Could you check a few things on this drawing? It's one solid part, dimensions in mm from its lowest x, y, z. A direction names the side the tool comes from. Give positions to 0.01 mm unless a question says otherwise; leave off trailing zeros. Loops run counter-clockwise (first coordinate to the right, second up) from the corner with the lowest first, then second, coordinate; pieces in that order, holes last. Notation, with made-up numbers: M 66.5,-10.5 L 92.5,-10.5 A22 cw 92.5,5.5 Z; hole C 49,83.25 d6. An arc over 180 degrees is marked long. One line per item, written item: value. Start each with the question number.
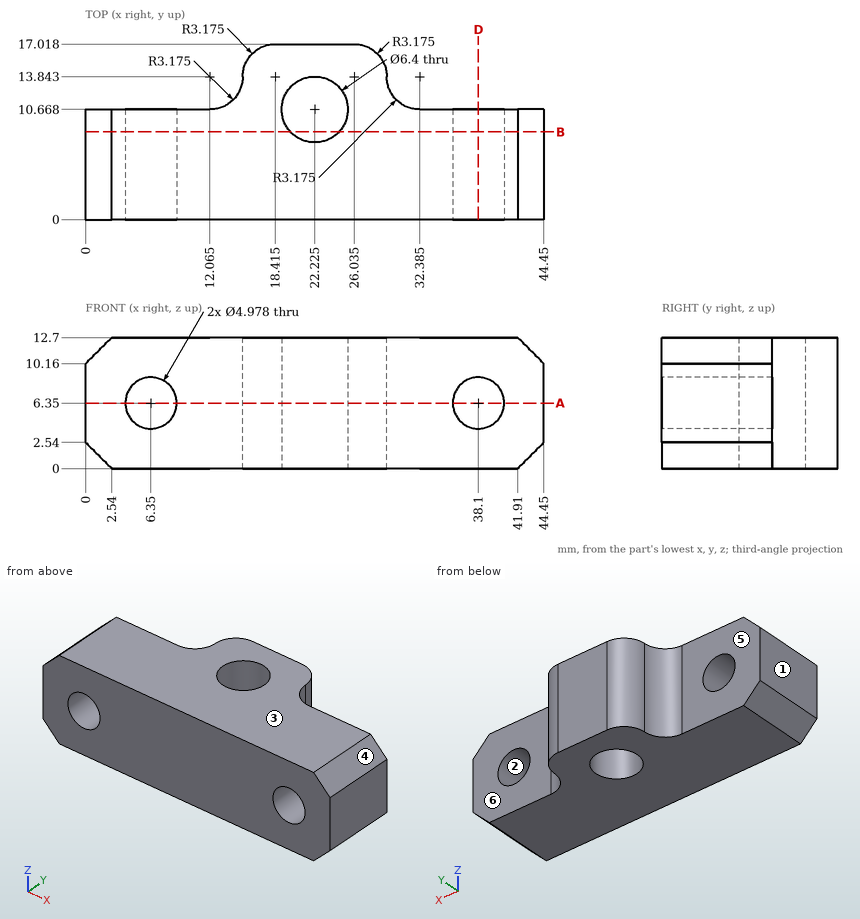
Q1. I need wall thicknesses on line 1 along Z through (x, y) = (6.35, 3); line 2 along X through (y, z) = (3, 7.25); line 3 along Y through (x, z) = (20, 5.5). Which ranges of each line are inside material? Lowest first, please.
Q2. If we section it at B-B, the plane y = 8.5: Write out the boundary of the cut face in (x, z), plus the area to 3 significant figures.
Q3. If we section it at A-A, the plane z = 6.35: Give the number of separate pieces and of enclosed holes in the cut face.
Q4. Which directions (+Z, -Z, +X, -X, +Y, -Y) give clear straight access to the entire face, cutting with the end or side of a thin tool? Please do the marked faces 4, 5 and 6.
Q5. If we mould it in two halves opening along X, with no side actions, what happens to the marked faces 1, 2 and 3? For each: released by +X, released by -X, zero draft, split by the parting line, or undercut.
Q6. For P1, Ø6, axis at x = 5.5, z = 5.5, coming from the +Y side, with a flat end and sliding along its axis, tell me the tip position at first contact or that it passes through.
Q7. If we section it at D-D, the plane x = 38.1: Write out the boundary of the cut face in (y, z).
Response:
1. line 1: 0 to 3.86, 8.84 to 12.7
1. line 2: 0 to 4.03, 8.67 to 35.78, 40.42 to 44.45
1. line 3: 0 to 8.37, 12.97 to 17.02
2. outline: M 0,2.54 L 2.54,0 L 19.87,0 L 19.87,12.7 L 2.54,12.7 L 0,10.16 Z; M 24.58,0 L 41.91,0 L 44.45,2.54 L 44.45,10.16 L 41.91,12.7 L 24.58,12.7 Z; hole C 6.35,6.35 d4.98; hole C 38.1,6.35 d4.98
2. area: 453 mm^2
3. separate pieces: 3
3. enclosed holes: 1
4. face 4: +Z, +X, +Y, -Y
4. face 5: +Z, -Z, -X, +Y
4. face 6: +Z, -Z, +X, +Y
5. face 1: released by -X
5. face 2: undercut
5. face 3: zero draft
6. P1: y = 10.67
7. outline: M 0,0 L 10.67,0 L 10.67,3.86 L 0,3.86 Z; M 0,8.84 L 10.67,8.84 L 10.67,12.7 L 0,12.7 Z
